The listing builds one solid part. Answer for the finished solid, in the listing's coordinates (mm). Face numbers are marked on the shaded views. Round coordinates to 2 decimals unless told otherwise and drop trailing zeros. Write each loop counter-clockwise with the first axis right and the second up, starting at its lowest first coordinate (ties: lowest second). Pieces come first, ordered by that corner, then holes. Notation, with made-up numbers: M -24,-6.5 L 33,-6.5 A18 cw 33,4.5 Z; hole C 28,-24 d11. An arc over 180 degrees is marked long. One line per item, written item: value. Start each with the question number.
(1) For a pull along X with two mould halves and no side action, classify the marked faces 1, 2 and 3 as released by +X, released by -X, zero draft, split by the parting line, or undercut.
(2) Section C-C (x = -29) is taken. Determine the outline of the cut face in (y, z).
(3) Consider probe 1 along X at (y, z) = (-1, 2.2); probe 2 along X at (y, z) = (-1.75, 2.3); probe 3 along Y at (x, z) = (-10.5, 1.1). Determine where each line is inside the solid, lowest interval first.
(4) Section A-A (x = 12.5) is taken. Determine the outline of the cut face in (y, z).
(5) Given P1, Ø1.1, axis at y = -1.5, z = 2.5, coming from the -X side; P2, Ø0.9, axis at y = 0, z = 2, coming from the +X side; P3, Ø6, axis at x = 4, y = 0, coming from the +Z side, each flat-ended and moving along its own axis, determine where each tip first touches the part or whether it passes through.
(6) Section B-B (y = 0.75) is taken. Determine the outline of the cut face in (x, z), plus the area to 3 significant figures.
(7) Section D-D (z = 2.45) is taken. Determine the outline of the cut face in (x, y), plus the area to 3 significant figures.
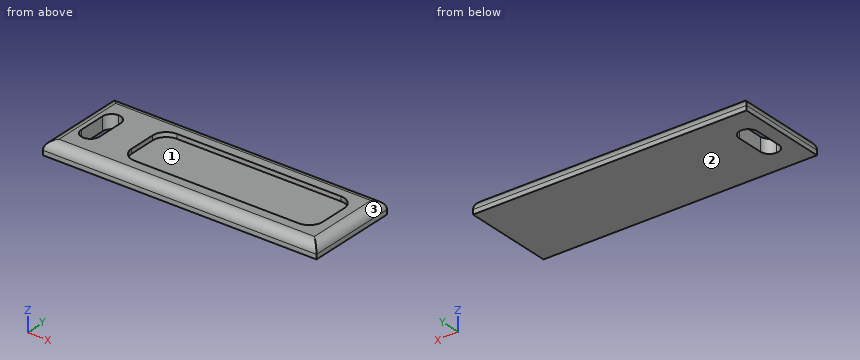
```python
from build123d import *

# Parameters (mm, degrees)
F0_W     = 50
F0_H     = 20
F0_W_2   = 10
F1_DEPTH = 3
F3_DEPTH = 3
F6_R     = 2


with BuildPart() as f1:
    # F0 (on Top) → F1 (new body)
    with BuildSketch(Plane.XY):
        Rectangle(F0_W, F0_H)
        with Locations((-30, 0)):
            Rectangle(F0_W_2, F0_H)
        with BuildLine():
            ThreePointArc((-30, 5), (-28.585786, 4.414214), (-28, 3))
            Line((-28, 3), (-28, -3))
            ThreePointArc((-28, -3), (-28.585786, -4.414214), (-30, -5))
            ThreePointArc((-30, -5), (-31.414214, -4.414214), (-32, -3))
            Line((-32, -3), (-32, 3))
            ThreePointArc((-32, 3), (-31.414214, 4.414214), (-30, 5))
        make_face(mode=Mode.SUBTRACT)
    extrude(amount=F1_DEPTH)


with BuildPart() as f3:
    # F2 (on Top) → F3 (new body)
    with BuildSketch(Plane.XY):
        with BuildLine():
            Line((-18, -6), (18, -6))
            ThreePointArc((18, -6), (20.12132, -5.12132), (21, -3))
            Line((21, -3), (21, 3))
            ThreePointArc((21, 3), (20.12132, 5.12132), (18, 6))
            Line((18, 6), (-18, 6))
            ThreePointArc((-18, 6), (-20.12132, 5.12132), (-21, 3))
            Line((-21, 3), (-21, -3))
            ThreePointArc((-21, -3), (-20.12132, -5.12132), (-18, -6))
        make_face()
    extrude(amount=F3_DEPTH)


with BuildPart() as f3_1:
    # F4: moved
    add(f3.part.moved(Location((0, 0, 2))))


with BuildPart() as f1_1:
    add(f1.part)

    # F5: cut F3
    add(f3_1.part, mode=Mode.SUBTRACT)

    # F6
    f6_edges = [f1_1.edges().sort_by_distance(p)[0] for p in [
        (-35, 0, 3),
        (25, 0, 3),
        (-5, 10, 3),
        (-5, -10, 3),
    ]]
    fillet(f6_edges, radius=F6_R)


solid = f1_1.part
```
Recorded:
1. face 1: undercut
1. face 2: zero draft
1. face 3: released by +X
2. outline: M -10,0 L -4.73,0 L -4.73,3 L -8,3 A2 ccw -10,1 Z; M 4.73,0 L 10,0 L 10,1 A2 ccw 8,3 L 4.73,3 Z
3. probe 1: x = -34.6 to -32, -28 to -21, 21 to 24.6
3. probe 2: x = -34.52 to -32, -28 to -21, 21 to 24.52
3. probe 3: y = -10 to 10
4. outline: M -10,0 L 10,0 L 10,1 A2 ccw 8,3 L 6,3 L 6,2 L -6,2 L -6,3 L -8,3 A2 ccw -10,1 Z
5. P1: stops at x = -34.76
5. P2: stops at x = 24.92
5. P3: stops at z = 2
6. outline: M -35,0 L -32,0 L -32,3 L -33,3 A2 ccw -35,1 Z; M -28,0 L 25,0 L 25,1 A2 ccw 23,3 L 21,3 L 21,2 L -21,2 L -21,3 L -28,3 Z
6. area: 124 mm2
7. outline: M -34.38,-9.38 L 24.38,-9.38 L 24.38,9.38 L -34.38,9.38 Z; hole M -32,-3 A2 ccw -30,-5 A2 ccw -28,-3 L -28,3 A2 ccw -30,5 A2 ccw -32,3 Z; hole M -21,-3 A3 ccw -18,-6 L 18,-6 A3 ccw 21,-3 L 21,3 A3 ccw 18,6 L -18,6 A3 ccw -21,3 Z
7. area: 569 mm2
